```python
from build123d import *

# Parameters (mm, degrees)
SKETCH_1_R           = 26
EXTRUDE_1_DEPTH      = 2
SKETCH_2_R           = 26
SKETCH_2_R_2         = 24
EXTRUDE_2_DEPTH      = 19
EXTRUDE_3_REACH      = 84.11
EXTRUDE_3_END_RADIUS = 26
SKETCH_4_W           = 25
SKETCH_4_H           = 12
SKETCH_5_W           = 25
SKETCH_5_H           = 20
CUT_EXTRUDE_1_DEPTH  = 6
EXTRUDE_5_REACH      = 67.759
CUT_EXTRUDE_START    = -19
SKETCH_7_R           = 24
CUT_EXTRUDE_2_DEPTH  = 19
EXTRUDE_START        = 5
SKETCH_8_R           = 24
EXTRUDE_6_DEPTH      = 5
FILLET_1_R           = 5


with BuildPart() as part:
    # Эскиз1 → Бобышка-Вытянуть1 (new body)
    with BuildSketch(Plane(origin=(0, 0, 0), x_dir=(1, 0, 0), z_dir=(0, 1, 0))):
        with Locations(Location((0, 0, 0), (0, 0, 270))):
            Circle(SKETCH_1_R)
    extrude(amount=EXTRUDE_1_DEPTH)

    # Эскиз2 → Бобышка-Вытянуть2 (add)
    with BuildSketch(Plane(origin=(0, 2, 0), x_dir=(1, 0, 0), z_dir=(0, 1, 0))):
        with Locations(Location((0, 0, 0), (0, 0, 270))):
            Circle(SKETCH_2_R)
        with Locations(Location((0, 0, 0), (0, 0, 270))):
            Circle(SKETCH_2_R_2, mode=Mode.SUBTRACT)
    extrude(amount=EXTRUDE_2_DEPTH)

    # Бобышка-Вытянуть3: up to this cylinder (the profile starts outside it)
    extrude_3_end = Plane(origin=(0, 6, 0), z_dir=(0, -1, 0)) * Cylinder(EXTRUDE_3_END_RADIUS, 221.22, mode=Mode.PRIVATE)
    # Эскиз4 → Бобышка-Вытянуть3 (add, up to the surface)
    with BuildSketch(Plane.XY.offset(49), mode=Mode.PRIVATE) as extrude_3_sk1:
        with Locations((0, 6)):
            Rectangle(SKETCH_4_W, SKETCH_4_H)
    extrude_3_tool1 = extrude(extrude_3_sk1.sketch, amount=-EXTRUDE_3_REACH, mode=Mode.PRIVATE) - extrude_3_end
    add(extrude_3_tool1.solids().sort_by_distance((0, 6, 49))[0])

    # Эскиз5 → Вырез-Вытянуть1 (cut)
    with BuildSketch(Plane.XZ):
        with Locations((0, 39)):
            Rectangle(SKETCH_5_W, SKETCH_5_H)
    extrude(amount=-CUT_EXTRUDE_1_DEPTH, mode=Mode.SUBTRACT)

    # Бобышка-Вытянуть5: up to this face of the body (flat: up to its plane)
    extrude_5_end = Plane(part.part.faces().sort_by_distance((-12.5, 7.851626254, 33.985056872))[0])
    # Эскиз6 → Бобышка-Вытянуть5 (add, up to the picked face)
    with BuildSketch(Plane(origin=(12.5, 0, 0), x_dir=(0, 0, -1), z_dir=(1, 0, 0)), mode=Mode.PRIVATE) as extrude_5_sk1:
        with BuildLine():
            Line((-26, 21), (-22.79802623, 21))
            Line((-22.79802623, 21), (-22.79802623, 12))
            Line((-22.79802623, 12), (-49, 12))
            add(Edge.make_bspline(
                [(-49, 12), (-38.341292939, 12), (-34.129850558, 21), (-26, 21)],
                knots=[0, 0, 0, 0, 1, 1, 1, 1], degree=3))
        make_face()
    extrude_5_tool1 = split(extrude(extrude_5_sk1.sketch, amount=-EXTRUDE_5_REACH, mode=Mode.PRIVATE), bisect_by=extrude_5_end, keep=Keep.BOTH, mode=Mode.PRIVATE)
    add(extrude_5_tool1.solids().sort_by(Axis((12.5, 15.609347, 30.602096), (-1, 0, 0)))[0])

    # Эскиз7 → Вырез-Вытянуть2 (cut)
    with BuildSketch(Plane(origin=(0, 21, 0), x_dir=(1, 0, 0), z_dir=(0, 1, 0)).offset(CUT_EXTRUDE_START)):
        with Locations(Location((0, 0, 0), (0, 0, 270))):
            Circle(SKETCH_7_R)
    extrude(amount=CUT_EXTRUDE_2_DEPTH, mode=Mode.SUBTRACT)

    # Эскиз8 → Бобышка-Вытянуть6 (add)
    with BuildSketch(Plane.XZ.offset(EXTRUDE_START)):
        with BuildLine():
            ThreePointArc((-12.5, 22.79802623), (0, -26), (12.5, 22.79802623))
            ThreePointArc((12.5, 22.79802623), (0, 26), (-12.5, 22.79802623))
        make_face()
        with Locations(Location((0, 0, 0), (0, 0, 90))):
            Circle(SKETCH_8_R, mode=Mode.SUBTRACT)
    extrude(amount=-EXTRUDE_6_DEPTH)

    # Скругление1
    fillet_1_edges = [part.edges().sort_by_distance(p)[0] for p in [
        (12.5, 10.5, 22.79802623),
        (-12.5, 10.5, 22.79802623),
    ]]
    fillet(fillet_1_edges, radius=FILLET_1_R)


solid = part.part
```
Check sheet for the modelled part. Datum: model origin and axes. Units: mm. A direction names the side the tool comes from. Round coordinates to 2 decimals unless told otherwise and drop trailing zeros. Order: outer loops, then holes, each group sorted by start corner. A loop starts at its lowest first (then second) coordinate and runs counter-clockwise, first axis right, second up. Notation, with made-up numbers: (-25.5, -6.5) - (26.5, -6.5) arc R21 ccw to (26.5, 4.5) - close; hole circle Ø4 at (71.25, 56). An arc over 180 degrees is marked (long way). Answer as CSV lines item,"result". Start each with the question number.
1) Section check C-C (x = 17). Record the cut outline in (y, z).
2) Section check A-A (y = 11). Record the cut outline in (x, z).
3) Depth check by flat-ended pin: pin 1 (6 mm diameter, centred on x = 3.5, z = 26, fed in from -Y); pin 2 (5 mm diameter, centred on x = 2.5, z = -3.5, fed in from -Y); pin 3 (2 mm diameter, centred on x = 10.5, z = 29, fed in from +Y); pin 4 (6 mm diameter, centred on x = 2.5, z = 39, fed in from -Y). Enter the tip coordinate at first touch or a pass-through.
4) Draft check along Z on faces 6 (the face through (0, 0, 0)), 7 (the face through (-13.094, 10.353, 23.225)), 8 (the face through (-11.4, 21, 21.3)). Enter one of: +Z half, -Z half, draft (parallel to the pull), parting line (faces both ways), or undercut.
5) Section check B-B (z = 0). Record the cut outline in (x, y), then the cut area to 3 significant figures.
6) Scan lines: probe 1 along X at (y, z) = (5.75, 0); probe 2 along Y at (x, z) = (-8.5, -19.5); probe 3 along Z at (x, y) = (-17, 9.5). Record each from-to range of solid material in increasing order.
7) Tool access check on faces 1 (the face through (7.21, 11.37, 22.89)), 2 (the face through (12.5, 11, 35)), 3 (the face through (-7.21, -2.54, 22.89)), 4 (the face through (0, 6, 39)), 5 (the face through (-12.5, 10, 35)). Record the directions out of +Z, -Z, +X, -X, +Y, -Y that give a thin tool (end or side, any length) a straight path to the whole face; none if there is none.
Determined:
1,outline,"(-5, -19.67) - (21, -19.67) - (21, -16.94) - (2, -16.94) - (2, 16.94) - (21, 16.94) - (21, 19.67) - (-5, 19.67) - (-5, 16.94) - (0, 16.94) - (0, -16.94) - (-5, -16.94) - close"
2,outline,"(-14.68, 21.46) arc R26 ccw (long way) to (14.68, 21.46) arc R5 cw to (12.5, 25.59) - (12.5, 49) - (-12.5, 49) - (-12.5, 25.59) arc R5 cw to start; hole circle Ø48 at (0, 0)"
3,pin 1,"y = -5"
3,pin 2,"y = 0"
3,pin 3,"y = 20.81"
3,pin 4,"y = 6"
4,face 6,"undercut"
4,face 7,"+Z half"
4,face 8,"draft"
5,outline,"(-26, -5) - (-24, -5) - (-24, 0) - (24, 0) - (24, -5) - (26, -5) - (26, 21) - (24, 21) - (24, 2) - (-24, 2) - (-24, 21) - (-26, 21) - close"
5,area,"200 mm^2"
6,probe 1,"-26 to -24, 24 to 26"
6,probe 2,"0 to 2"
6,probe 3,"-19.67 to -16.94, 16.94 to 19.67"
7,face 1,"+Y"
7,face 2,"+Z, +X, +Y, -Y"
7,face 3,"-Y"
7,face 4,"+Z, +X, -X, -Y"
7,face 5,"+Z, -X, +Y, -Y"
